Read the model definition and answer for the solid it produces. Units are mm, in the model's axes. Face numbers are marked on the shaded views. A direction names the side the tool comes from. Coordinates: 2 decimals unless noted, no trailing zeros. Write each loop counter-clockwise with the first axis right and the second up, starting at its lowest first coordinate (ties: lowest second). Pieces come first, ordered by that corner, then holes. Notation, with made-up numbers: (19.25, 24) -> (32.25, 24) arc R16 ccw to (32.25, 41) -> close; hole circle Ø1 at (74.5, 65). An arc over 180 degrees is marked (long way). One line per item, written item: value. Start each with the question number.
1. Find section D-D, the plane x = -6. Write down the section's boundary in (y, z), and give its area (3 significant figures).
2. Find section C-C, the plane z = 16.5. Write down the section's boundary in (x, y) (1 decimal).
3. For the marked faces 1 and 2, determine the directions among +Z, -Z, +X, -X, +Y, -Y from which every point of the face is accessible in a straight line to the end or side of a thin tool.
4. Consider line 1 along Y through (x, z) = (-1.25, 27); line 2 along Z through (x, y) = (-2.5, -4.75); line 3 along Z through (x, y) = (2, -2.25). Determine where each line is inside the solid, lowest interval first.
5. Given P1, Ø1, axis at x = -4, z = 29.5, coming from the +Y side; P2, Ø6, axis at x = 5, y = -2, coming from the +Z side; P3, Ø6, axis at y = 4, z = 20.5, coming from the -X side; P4, Ø1, axis at y = 0, z = 17, coming from the +X side, each flat-ended and moving along its own axis, determine where each tip first touches the part or whether it passes through.
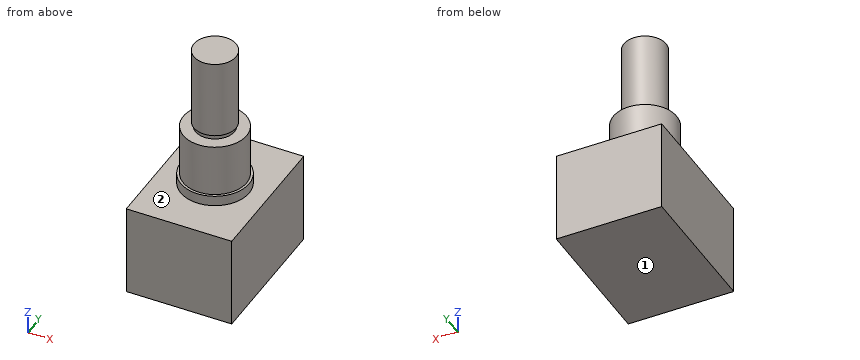
```python
from build123d import *

# Parameters (mm, degrees)
SKETCH1_W           = 15.875
SKETCH1_H           = 21.209
BOSS_EXTRUDE1_DEPTH = 13.8938
SKETCH2_R           = 5.1435
BOSS_EXTRUDE2_DEPTH = 1.5748
SKETCH3_R           = 4.7625
BOSS_EXTRUDE3_DEPTH = 9.525
SKETCH4_R           = 3.175
BOSS_EXTRUDE4_DEPTH = 22.225
SKETCH5_W           = 0.254
SKETCH5_H           = 0.7366


with BuildPart() as part:
    # Sketch1 → Boss-Extrude1 (new body)
    with BuildSketch(Plane.XY):
        Rectangle(SKETCH1_W, SKETCH1_H)
    extrude(amount=BOSS_EXTRUDE1_DEPTH)

    # Sketch2 → Boss-Extrude2 (add)
    with BuildSketch(Plane.XY.offset(13.8938)):
        Circle(SKETCH2_R)
    extrude(amount=BOSS_EXTRUDE2_DEPTH)

    # Sketch3 → Boss-Extrude3 (add)
    with BuildSketch(Plane.XY.offset(13.8938)):
        Circle(SKETCH3_R)
    extrude(amount=BOSS_EXTRUDE3_DEPTH)

    # Sketch4 → Boss-Extrude4 (add)
    with BuildSketch(Plane.XY.offset(13.8938)):
        Circle(SKETCH4_R)
    extrude(amount=BOSS_EXTRUDE4_DEPTH)

    # Sketch5 → Cut-Revolve1 (revolve, cut)
    with BuildSketch(Plane(origin=(0, 0, 0), x_dir=(1, 0, 0), z_dir=(0, 1, 0))):
        with Locations((3.048, -23.7871)):
            Rectangle(SKETCH5_W, SKETCH5_H)
    revolve(axis=Axis((0, 0, 36.1188), (0, 0, -1)), mode=Mode.SUBTRACT)


solid = part.part
```
Answer block:
1. outline: (-10.6, 0) -> (10.6, 0) -> (10.6, 13.89) -> (-10.6, 13.89) -> close
1. area: 295 mm2
2. outline: circle Ø9.5 at (0, 0)
3. face 1: -Z, +X, -X, +Y, -Y
3. face 2: +Z
4. line 1: y = -2.92 to 2.92
4. line 2: z = 0 to 13.89
4. line 3: z = 0 to 23.42, 24.16 to 36.12
5. P1: passes through
5. P2: stops at z = 36.12
5. P3: stops at x = -4.66
5. P4: stops at x = 4.76
